```python
from build123d import *

# Parameters (mm, degrees)
BOSS_EXTRUDE1_DEPTH = 25.4
CUT_EXTRUDE1_REACH  = 27.4
SKETCH2_R           = 4
SKETCH2_R_2         = 0.79375
SKETCH3_W           = 3.175
SKETCH3_H           = 1.5875
CUT_EXTRUDE2_DEPTH  = 26.4
SKETCH4_R           = 10.99185
CUT_EXTRUDE3_DEPTH  = 6.985
SKETCH5_R           = 4.5
CUT_EXTRUDE4_DEPTH  = 19.415


with BuildPart() as part:
    # Sketch1 → Boss-Extrude1 (new body)
    with BuildSketch(Plane.XY):
        with BuildLine():
            Line((12.7, 50.8), (12.7, -50.8))
            ThreePointArc((12.7, -50.8), (0, -63.5), (-12.7, -50.8))
            Line((-12.7, -50.8), (-12.7, 50.8))
            ThreePointArc((-12.7, 50.8), (0, 63.5), (12.7, 50.8))
        make_face()
    extrude(amount=BOSS_EXTRUDE1_DEPTH)

    # Sketch2 → Cut-Extrude1 (cut, up to next)
    with BuildSketch(Plane.XY.offset(25.4), mode=Mode.PRIVATE) as cut_extrude1_sk1:
        with Locations((0, 50.8)):
            Circle(SKETCH2_R)
    cut_extrude1_tool1 = extrude(cut_extrude1_sk1.sketch, amount=-CUT_EXTRUDE1_REACH, mode=Mode.PRIVATE) & part.part
    add(cut_extrude1_tool1.solids().sort_by_distance((0, 50.8, 25.4))[0], mode=Mode.SUBTRACT)
    # Sketch2 → Cut-Extrude1 (cut, up to next)
    with BuildSketch(Plane.XY.offset(25.4), mode=Mode.PRIVATE) as cut_extrude1_sk2:
        with Locations((-4.939140867, 55.739140867)):
            Circle(SKETCH2_R_2)
    cut_extrude1_tool2 = extrude(cut_extrude1_sk2.sketch, amount=-CUT_EXTRUDE1_REACH, mode=Mode.PRIVATE) & part.part
    add(cut_extrude1_tool2.solids().sort_by_distance((-4.939141, 55.739141, 25.4))[0], mode=Mode.SUBTRACT)
    # Sketch2 → Cut-Extrude1 (cut, up to next)
    with BuildSketch(Plane.XY.offset(25.4), mode=Mode.PRIVATE) as cut_extrude1_sk3:
        with Locations((-4.939140867, 45.860859133)):
            Circle(SKETCH2_R_2)
    cut_extrude1_tool3 = extrude(cut_extrude1_sk3.sketch, amount=-CUT_EXTRUDE1_REACH, mode=Mode.PRIVATE) & part.part
    add(cut_extrude1_tool3.solids().sort_by_distance((-4.939141, 45.860859, 25.4))[0], mode=Mode.SUBTRACT)
    # Sketch2 → Cut-Extrude1 (cut, up to next)
    with BuildSketch(Plane.XY.offset(25.4), mode=Mode.PRIVATE) as cut_extrude1_sk4:
        with Locations((4.939140867, 55.739140867)):
            Circle(SKETCH2_R_2)
    cut_extrude1_tool4 = extrude(cut_extrude1_sk4.sketch, amount=-CUT_EXTRUDE1_REACH, mode=Mode.PRIVATE) & part.part
    add(cut_extrude1_tool4.solids().sort_by_distance((4.939141, 55.739141, 25.4))[0], mode=Mode.SUBTRACT)
    # Sketch2 → Cut-Extrude1 (cut, up to next)
    with BuildSketch(Plane.XY.offset(25.4), mode=Mode.PRIVATE) as cut_extrude1_sk5:
        with Locations((4.939140867, 45.860859133)):
            Circle(SKETCH2_R_2)
    cut_extrude1_tool5 = extrude(cut_extrude1_sk5.sketch, amount=-CUT_EXTRUDE1_REACH, mode=Mode.PRIVATE) & part.part
    add(cut_extrude1_tool5.solids().sort_by_distance((4.939141, 45.860859, 25.4))[0], mode=Mode.SUBTRACT)

    # Sketch3 → Cut-Extrude2 (cut, through all)
    with BuildSketch(Plane.XY.offset(25.4)):
        with Locations((0, 55.265240671)):
            Rectangle(SKETCH3_W, SKETCH3_H)
    extrude(amount=-CUT_EXTRUDE2_DEPTH, mode=Mode.SUBTRACT)

    # Sketch4 → Cut-Extrude3 (cut)
    with BuildSketch(Plane.XY.offset(25.4)):
        with Locations((0, -50.8)):
            Circle(SKETCH4_R)
    cut_extrude3 = extrude(amount=-CUT_EXTRUDE3_DEPTH, mode=Mode.SUBTRACT)

    # Mirror1: Cut-Extrude3 across plane
    add(cut_extrude3.mirror(Plane.XY.offset(12.7)), mode=Mode.SUBTRACT)

    # Sketch5 → Cut-Extrude4 (cut, through all)
    with BuildSketch(Plane.XY.offset(18.415)):
        with Locations((0, -50.8)):
            Circle(SKETCH5_R)
    extrude(amount=-CUT_EXTRUDE4_DEPTH, mode=Mode.SUBTRACT)


solid = part.part
```
Model file for the job. Use its own axes, mm. A direction names the side the tool comes from. Give positions to 0.01 mm unless a question says otherwise; leave off trailing zeros. Write each loop counter-clockwise with the first axis right and the second up, starting at its lowest first coordinate (ties: lowest second). Pieces come first, ordered by that corner, then holes. Notation, with made-up numbers: (1, 41.5) - (22, 41.5) arc R31 cw to (22, 71.5) - close; hole circle Ø5 at (26.25, 64). An arc over 180 degrees is marked (long way). One line per question, with ' | ' between items. Start each with the question number.
(1) Slice it at B-B on z = 9.75. Write the cut outline in (x, y).
(2) Slice it at C-C on x = -7.25. Write the cut outline in (y, z) (3 decimals).
(3) 3-axis set-ups, long thin cutter, end or side, ignore diameter. For faces 1 (the face through (0, -56, 6.985)), 2 (the face through (0, 56.059, 13)), 3 (the face through (5.072, -60.552, 21.956)): which of +Z, -Z, +X, -X, +Y, -Y reach the whole face in a straight line?
(4) Slice it at D-D on y = -42.5. Write the cut outline in (x, z) (3 decimals).
(5) Pin check, flat tips, straight feed: P1, Ø10, axis at x = -7.5, z = 21.5, coming from the +Y side; P2, Ø1.7, axis at y = 55, z = 12, coming from the -X side; P3, Ø11, axis at x = 0, y = -48.5, coming from the +Z side (3 decimals). Stop position of each tip, or through.
(6) Slice it at A-A on x = 0. Write the cut outline in (y, z) (3 decimals), plus the area to 3 significant figures.
(7) Two-plate mould, pull along Y, no slides. Class faces 4 (the face through (-12.7, -1, 13)), 5 (the face through (0, -56, 18.415)), 6 (the face through (-0.279, 63.497, 12.522)): +Y half, -Y half, draft (parallel to the pull), parting line (faces both ways), or undercut.
(8) Wall check: line 1 along Y through (x, z) = (0, 20.25); line 2 along Y through (x, z) = (0, 15.75); line 3 along X through (y, z) = (50.8, 11). Give the ranges that are in metal, low to high. Write a range as from..to.
Results below:
1) outline: (-12.7, -50.8) arc R12.7 ccw to (12.7, -50.8) - (12.7, 50.8) arc R12.7 ccw to (-12.7, 50.8) - close; hole circle Ø1.59 at (-4.94, 45.86); hole circle Ø1.59 at (-4.94, 55.74); hole circle Ø9 at (0, -50.8); hole (-1.59, 54.47) arc R4 ccw (long way) to (1.59, 54.47) - (1.59, 56.06) - (-1.59, 56.06) - close; hole circle Ø1.59 at (4.94, 45.86); hole circle Ø1.59 at (4.94, 55.74)
2) outline: (-61.227, 0) - (-59.062, 0) - (-59.062, 6.985) - (-42.538, 6.985) - (-42.538, 0) - (61.227, 0) - (61.227, 25.4) - (-42.538, 25.4) - (-42.538, 18.415) - (-59.062, 18.415) - (-59.062, 25.4) - (-61.227, 25.4) - close
3) face 1: -Z | face 2: +Z, -Z | face 3: +Z
4) outline: (-12.7, 0) - (-7.206, 0) - (-7.206, 6.985) - (7.206, 6.985) - (7.206, 0) - (12.7, 0) - (12.7, 25.4) - (7.206, 25.4) - (7.206, 18.415) - (-7.206, 18.415) - (-7.206, 25.4) - (-12.7, 25.4) - close
5) P1: y = 63.25 | P2: x = -12.25 | P3: z = 18.415
6) outline: (-63.5, 0) - (-61.792, 0) - (-61.792, 6.985) - (-55.3, 6.985) - (-55.3, 18.415) - (-61.792, 18.415) - (-61.792, 25.4) - (-63.5, 25.4) - close; (-46.3, 6.985) - (-39.808, 6.985) - (-39.808, 0) - (46.8, 0) - (46.8, 25.4) - (-39.808, 25.4) - (-39.808, 18.415) - (-46.3, 18.415) - close; (56.059, 0) - (63.5, 0) - (63.5, 25.4) - (56.059, 25.4) - close | area: 2,580 mm^2
7) face 4: draft | face 5: undercut | face 6: +Y half
8) line 1: -63.5..-61.79, -39.81..46.8, 56.06..63.5 | line 2: -63.5..-55.3, -46.3..46.8, 56.06..63.5 | line 3: -12.7..-4, 4..12.7
